Autodesk Inventor part; units mm, degrees
ref_plane "YZ Plane" through (0, 0, 0) normal (1, 0, 0) x (0, 1, 0)
ref_plane "XZ Plane" through (0, 0, 0) normal (0, 1, 0) x (-1, 0, 0)
ref_plane "XY Plane" through (0, 0, 0) normal (0, 0, 1) x (1, 0, 0)
sketch "Sketch2" plane through (0, 0, 0) normal (0, 1, 0) x (-1, 0, 0)
  line L0 (0, 0) -> (177.8, 0)
  line L1 (177.8, 0) -> (177.8, 228.6)
  line L2 (177.8, 228.6) -> (0, 228.6)
  line L3 (0, 228.6) -> (0, 0)
  dimension "d0" = 177.8
  dimension "d1" = 228.6
extrude "Extrusion1" add sketch "Sketch2" along normal blind 6.35
sketch "Sketch3" plane through (0, 6.35, 0) normal (0, 1, 0) x (1, 0, 0)
  line L0 (-177.8, -228.6) -> (0, -228.6)
  line L1 (-177.8, 0) -> (-177.8, -228.6)
  line L2 (0, 0) -> (-177.8, 0)
  line L3 (0, -228.6) -> (0, 0)
  line L4 (-88.9, -228.6) -> (-88.9, -222.25) construction
  line L5 (-88.9, 0) -> (-88.9, -6.35) construction
  line L6 (-177.8, -114.3) -> (-171.45, -114.3) construction
  line L7 (0, -114.3) -> (-6.35, -114.3) construction
  line L8 (-171.45, -114.3) -> (-171.45, -6.35)
  line L9 (-171.45, -114.3) -> (-171.45, -222.25)
  line L10 (-171.45, -6.35) -> (-88.9, -6.35)
  line L11 (-6.35, -6.35) -> (-88.9, -6.35)
  line L12 (-6.35, -6.35) -> (-6.35, -114.3)
  line L13 (-6.35, -114.3) -> (-6.35, -222.25)
  line L14 (-6.35, -222.25) -> (-88.9, -222.25)
  line L15 (-171.45, -222.25) -> (-88.9, -222.25)
  line L16 (-177.8, -228.6) -> (0, -228.6)
  line L17 (0, -228.6) -> (0, 0)
  line L18 (0, 0) -> (-177.8, 0)
  line L19 (-177.8, 0) -> (-177.8, -228.6)
  dimension "d4" = 6.35
  dimension "d5" = 6.35
  dimension "d6" = 6.35
  dimension "d7" = 6.35
extrude "Extrusion2" add sketch "Sketch3" along normal blind 38.1
sketch "Sketch4" plane through (0, 0, 0) normal (0, -1, 0) x (1, 0, 0)
  line L0 (-177.8, 0) -> (-177.8, 228.6)
  line L1 (-177.8, 228.6) -> (0, 228.6) construction
  line L2 (0, 228.6) -> (0, 0)
  line L3 (0, 0) -> (-177.8, 0)
  line L4 (-88.9, 228.6) -> (-88.9, 0) construction
  line L5 (0, 114.3) -> (-177.8, 114.3) construction
  line L6 (-88.9, 228.6) -> (-68.58, 228.6)
  line L7 (0, 228.6) -> (-177.8, 228.6) construction
  line L8 (-88.9, 228.6) -> (-109.22, 228.6)
  line L9 (-68.58, 228.6) -> (-68.58, 0) construction
  line L10 (-109.22, 228.6) -> (-109.22, 0) construction
  line L11 (-68.58, 228.6) -> (-68.58, 177.8) construction
  line L12 (-109.22, 228.6) -> (-109.22, 177.8) construction
  line L13 (-68.58, 177.8) -> (-68.58, 187.325) construction
  line L14 (-68.58, 177.8) -> (-68.58, 168.275) construction
  circle A0 centre (-68.58, 187.325) radius 2.413
  circle A1 centre (-68.58, 168.275) radius 2.413
  line L15 (-68.58, 187.325) -> (0, 187.325) construction
  line L16 (0, 187.325) -> (-12.7, 187.325) construction
  line L17 (-68.58, 168.275) -> (0, 168.275) construction
  line L18 (0, 168.275) -> (-12.7, 168.275) construction
  circle A2 centre (-12.7, 187.325) radius 2.413
  circle A3 centre (-12.7, 168.275) radius 2.413
  circle A4 centre (-68.58, 215.9) radius 2.413
  circle A5 centre (-109.22, 187.325) radius 2.413
  circle A6 centre (-109.22, 168.275) radius 2.413
  circle A7 centre (-165.1, 187.325) radius 2.413
  circle A8 centre (-165.1, 168.275) radius 2.413
  circle A9 centre (-109.22, 215.9) radius 2.413
  circle A10 centre (-68.58, 41.275) radius 2.413
  circle A11 centre (-68.58, 60.325) radius 2.413
  circle A12 centre (-12.7, 41.275) radius 2.413
  circle A13 centre (-12.7, 60.325) radius 2.413
  circle A14 centre (-68.58, 12.7) radius 2.413
  circle A15 centre (-109.22, 12.7) radius 2.413
  circle A16 centre (-109.22, 41.275) radius 2.413
  circle A17 centre (-165.1, 41.275) radius 2.413
  circle A18 centre (-165.1, 60.325) radius 2.413
  circle A19 centre (-109.22, 60.325) radius 2.413
  dimension "d10" = 20.32
  dimension "d11" = 50.8
  dimension "d12" = 9.525
  dimension "d13" = 4.826
  dimension "d14" = 4.826
  dimension "d16" = 12.7
  dimension "d17" = 4.826
  dimension "d18" = 4.826
  dimension "d19" = 12.7
  dimension "d20" = 4.826
  dimension "d21" = 12.7
extrude "Extrusion3" cut sketch "Sketch4" against normal through all
sketch "Sketch5" plane through (0, 6.35, 0) normal (0, 1, 0) x (1, 0, 0)
  circle A0 centre (-109.22, -187.325) radius 2.413
  circle A1 centre (-68.58, -168.275) radius 2.413
  circle A2 centre (-12.7, -60.325) radius 2.413
  circle A3 centre (-68.58, -12.7) radius 2.413
  circle A4 centre (-165.1, -60.325) radius 2.413
  circle A5 centre (-109.22, -60.325) radius 2.413
  circle A6 centre (-68.58, -60.325) radius 2.413
  circle A7 centre (-12.7, -168.275) radius 2.413
  circle A8 centre (-109.22, -168.275) radius 2.413
  circle A9 centre (-109.22, -215.9) radius 2.413
  circle A10 centre (-165.1, -187.325) radius 2.413
  circle A11 centre (-68.58, -187.325) radius 2.413
  circle A12 centre (-12.7, -41.275) radius 2.413
  circle A13 centre (-109.22, -12.7) radius 2.413
  circle A14 centre (-165.1, -41.275) radius 2.413
  circle A15 centre (-109.22, -41.275) radius 2.413
  circle A16 centre (-68.58, -41.275) radius 2.413
  circle A17 centre (-12.7, -187.325) radius 2.413
  circle A18 centre (-165.1, -168.275) radius 2.413
  circle A19 centre (-68.58, -215.9) radius 2.413
  line L0 (-171.45, -222.25) -> (-6.35, -222.25)
  line L1 (-6.35, -222.25) -> (-6.35, -6.35)
  line L2 (-6.35, -6.35) -> (-171.45, -6.35)
  line L3 (-171.45, -6.35) -> (-171.45, -222.25)
  line L4 (-171.45, -114.3) -> (-6.35, -114.3) construction
  line L5 (-88.9, -6.35) -> (-88.9, -222.25) construction
  line L6 (-34.925, -168.275) -> (-142.875, -168.275) construction
  line L7 (-142.875, -168.275) -> (-142.875, -60.325) construction
  line L8 (-142.875, -60.325) -> (-34.925, -60.325) construction
  line L9 (-34.925, -60.325) -> (-34.925, -168.275) construction
  line L10 (-34.925, -168.275) -> (-142.875, -60.325) construction
  line L11 (-142.875, -168.275) -> (-34.925, -60.325) construction
  circle A20 centre (-88.9, -168.275) radius 2.413
  circle A21 centre (-142.875, -114.3) radius 2.413
  circle A22 centre (-88.9, -60.325) radius 2.413
  circle A23 centre (-34.925, -114.3) radius 2.413
  point P0 (0, 0)
  point P1 (-88.9, -114.3)
  dimension "d24" = 107.95
  dimension "d25" = 107.95
  dimension "d26" = 4.826
  dimension "d27" = 4.826
  dimension "d28" = 4.826
  dimension "d29" = 4.826
extrude "Extrusion4" cut sketch "Sketch5" against normal blind 6.35 contours A20 | A21 | A22 | A23
sketch "Sketch8" plane through (0, 6.35, 0) normal (0, 1, 0) x (1, 0, 0)
  circle A0 centre (-88.9, -168.275) radius 2.413
  circle A1 centre (-88.9, -60.325) radius 2.413
  circle A2 centre (-34.925, -114.3) radius 2.413
  circle A3 centre (-142.875, -114.3) radius 2.413
  circle A4 centre (-109.22, -187.325) radius 2.413
  circle A5 centre (-68.58, -168.275) radius 2.413
  circle A6 centre (-12.7, -60.325) radius 2.413
  circle A7 centre (-68.58, -12.7) radius 2.413
  circle A8 centre (-165.1, -60.325) radius 2.413
  circle A9 centre (-109.22, -60.325) radius 2.413
  circle A10 centre (-68.58, -60.325) radius 2.413
  circle A11 centre (-12.7, -168.275) radius 2.413
  circle A12 centre (-109.22, -168.275) radius 2.413
  circle A13 centre (-109.22, -215.9) radius 2.413
  circle A14 centre (-165.1, -187.325) radius 2.413
  circle A15 centre (-68.58, -187.325) radius 2.413
  circle A16 centre (-12.7, -41.275) radius 2.413
  circle A17 centre (-109.22, -12.7) radius 2.413
  circle A18 centre (-165.1, -41.275) radius 2.413
  circle A19 centre (-109.22, -41.275) radius 2.413
  circle A20 centre (-68.58, -41.275) radius 2.413
  circle A21 centre (-12.7, -187.325) radius 2.413
  circle A22 centre (-165.1, -168.275) radius 2.413
  circle A23 centre (-68.58, -215.9) radius 2.413
  line L0 (-171.45, -222.25) -> (-6.35, -222.25)
  line L1 (-6.35, -222.25) -> (-6.35, -6.35)
  line L2 (-6.35, -6.35) -> (-171.45, -6.35)
  line L3 (-171.45, -6.35) -> (-171.45, -222.25)
  line L4 (-142.875, -114.3) -> (-34.925, -114.3) construction
  line L5 (-88.9, -60.325) -> (-88.9, -168.275) construction
  line L6 (-114.3, -88.9) -> (-63.5, -88.9) construction
  line L7 (-63.5, -88.9) -> (-63.5, -139.7) construction
  line L8 (-63.5, -139.7) -> (-114.3, -139.7) construction
  line L9 (-114.3, -139.7) -> (-114.3, -88.9) construction
  line L10 (-114.3, -88.9) -> (-63.5, -139.7) construction
  line L11 (-63.5, -88.9) -> (-114.3, -139.7) construction
  circle A24 centre (-114.3, -88.9) radius 2.413
  circle A25 centre (-63.5, -88.9) radius 2.413
  circle A26 centre (-114.3, -139.7) radius 2.413
  circle A27 centre (-63.5, -139.7) radius 2.413
  point P0 (0, 0)
  point P1 (-88.9, -114.3)
  dimension "d38" = 50.8
  dimension "d39" = 50.8
  dimension "d40" = 4.826
  dimension "d41" = 4.826
  dimension "d42" = 4.826
  dimension "d43" = 4.826
extrude "Extrusion7" cut sketch "Sketch8" against normal through all contours A24 | A25 | A26 | A27
sketch "Sketch9" plane through (-177.8, 0, 228.6) normal (0, 0, 1) x (1, 0, 0)
  line L0 (177.8, 44.45) -> (0, 44.45)
  line L1 (88.9, 44.45) -> (88.9, 0) construction
  line L2 (91.313, 0) -> (86.487, 0)
  line L3 (177.8, 0) -> (177.8, 44.45)
  line L4 (0, 0) -> (0, 44.45)
  line L5 (177.8, 22.225) -> (0, 22.225) construction
  line L6 (67.31, 9.525) -> (110.49, 9.525)
  line L7 (110.49, 9.525) -> (110.49, 34.925)
  line L8 (110.49, 34.925) -> (67.31, 34.925)
  line L9 (67.31, 34.925) -> (67.31, 9.525)
  line L10 (67.31, 9.525) -> (110.49, 34.925) construction
  line L11 (110.49, 9.525) -> (67.31, 34.925) construction
  point P0 (88.9, 22.225)
  dimension "d46" = 43.18
  dimension "d47" = 25.4
extrude "Extrusion8" cut sketch "Sketch9" against normal through all
sketch "Sketch10" plane through (0, 0, 228.6) normal (1, 0, 0) x (0, 0, -1)
  line L0 (0, 0) -> (228.6, 0)
  line L1 (228.6, 0) -> (228.6, 44.45)
  line L2 (0, 44.45) -> (228.6, 44.45)
  line L3 (0, 0) -> (0, 44.45)
  line L4 (0, 22.225) -> (228.6, 22.225) construction
  line L5 (114.3, 44.45) -> (114.3, 0) construction
  line L6 (92.71, 9.525) -> (135.89, 9.525)
  line L7 (135.89, 9.525) -> (135.89, 34.925)
  line L8 (135.89, 34.925) -> (92.71, 34.925)
  line L9 (92.71, 34.925) -> (92.71, 9.525)
  line L10 (92.71, 9.525) -> (135.89, 34.925) construction
  line L11 (135.89, 9.525) -> (92.71, 34.925) construction
  point P0 (114.3, 22.225)
  dimension "d50" = 43.18
  dimension "d51" = 25.4
extrude "Extrusion9" cut sketch "Sketch10" against normal through all contours L9 L8 L7 L6
sketch "Sketch11" plane through (-177.8, 0, 228.6) normal (0, 0, 1) x (1, 0, 0)
  line L0 (67.31, 34.925) -> (110.49, 34.925)
  line L1 (110.49, 34.925) -> (110.49, 9.525)
  line L2 (110.49, 9.525) -> (67.31, 9.525)
  line L3 (67.31, 9.525) -> (67.31, 34.925)
  line L4 (0, 0) -> (177.8, 0)
  line L5 (177.8, 0) -> (177.8, 44.45)
  line L6 (0, 44.45) -> (177.8, 44.45)
  line L7 (0, 0) -> (0, 44.45)
  point P0 (177.8, 0)
extrude "Extrusion10" add sketch "Sketch11" along normal blind 2.54
sketch "Sketch12" plane through (0, 0, 0) normal (1, 0, 0) x (0, 0, -1)
  line L0 (-135.89, 34.925) -> (-92.71, 34.925)
  line L1 (-92.71, 34.925) -> (-92.71, 9.525)
  line L2 (-92.71, 9.525) -> (-135.89, 9.525)
  line L3 (-135.89, 9.525) -> (-135.89, 34.925)
  line L4 (0, 0) -> (-231.14, 0)
  line L5 (0, 0) -> (0, 44.45)
  line L6 (0, 44.45) -> (-231.14, 44.45)
  line L7 (-231.14, 0) -> (-231.14, 44.45)
  line L8 (0, 34.925) -> (0, 9.525)
  line L9 (0, 9.525) -> (0, 34.925)
  line L10 (0, 0) -> (0, 44.45)
  line L11 (0, 0) -> (0, 44.45)
extrude "Extrusion11" add sketch "Sketch12" along normal blind 2.54
sketch "Sketch13" plane through (-177.8, 0, 0) normal (0, 0, -1) x (-1, 0, 0)
  line L0 (-110.49, 34.925) -> (-67.31, 34.925)
  line L1 (-67.31, 34.925) -> (-67.31, 9.525)
  line L2 (-67.31, 9.525) -> (-110.49, 9.525)
  line L3 (-110.49, 9.525) -> (-110.49, 34.925)
  line L4 (0, 0) -> (-180.34, 0)
  line L5 (0, 0) -> (0, 44.45)
  line L6 (0, 44.45) -> (-180.34, 44.45)
  line L7 (-180.34, 0) -> (-180.34, 44.45)
  point P0 (-177.8, 0)
extrude "Extrusion12" add sketch "Sketch13" along normal blind 2.54
sketch "Sketch14" plane through (-177.8, 0, 231.14) normal (-1, 0, 0) x (0, 0, 1)
  line L0 (-138.43, 34.925) -> (-95.25, 34.925)
  line L1 (-95.25, 34.925) -> (-95.25, 9.525)
  line L2 (-95.25, 9.525) -> (-138.43, 9.525)
  line L3 (-138.43, 9.525) -> (-138.43, 34.925)
  line L4 (-233.68, 0) -> (0, 0)
  line L5 (0, 44.45) -> (0, 0)
  line L6 (0, 44.45) -> (-233.68, 44.45)
  line L7 (-233.68, 0) -> (-233.68, 44.45)
  point P0 (-231.14, 0)
extrude "Extrusion13" add sketch "Sketch14" along normal blind 2.54
fillet "Fillet1" radius 5.08 1 edges at (-180.34, 22.225, 231.14)
fillet "Fillet2" radius 5.08 1 edges at (2.54, 22.225, -2.54)
fillet "Fillet3" radius 5.08 1 edges at (2.54, 22.225, 231.14)
fillet "Fillet4" radius 5.08 1 edges at (-180.34, 22.225, -2.54)
fillet "Fillet5" radius 3.175 4 edges at (-88.9, 44.45, -2.54) (2.54, 44.45, 114.3) (-88.9, 44.45, 231.14) (-180.34, 44.45, 114.3)
equation "\"d2\" = base_thickness"
equation "\"d4\" = base_thickness"
equation "\"d5\" = base_thickness"
equation "\"d6\" = base_thickness"
equation "\"d7\" = base_thickness"
equation "\"d10\" = motor_adapter_across"
equation "\"d12\" = 0.5 * motor_adapter_width"
equation "\"d19\" = d16"
equation "\"d21\" = d16"
equation "\"base_thickness\" = 6.35"
equation "\"motor_adapter_width\" = 19.05"
equation "\"motor_adapter_across\" = 20.32"
properties part number "base"
Source: CAD feature listing. Evaluate the final solid. Frame: model axes, mm. A direction names the side the tool comes from. Round coordinates to 2 decimals unless told otherwise and drop trailing zeros. Loops run counter-clockwise (first coordinate to the right, second up) from the corner with the lowest first, then second, coordinate; pieces in that order, holes last. Notation, with made-up numbers: (-24.5, -8.75) -> (20.5, -8.75) arc R14 cw to (20.5, -1.75) -> close; hole circle Ø10 at (55.5, 63.25). An arc over 180 degrees is marked (long way). Answer as a JSON object with one key per item and string values. Group by question number.
Q1. Section query B-B (z = 114.3). Output: boundary loops of the cut face in (x, y) (3 decimals).
Q2. Section query A-A (x = -12.7). Output: boundary loops of the cut face in (y, z) (3 decimals), plus the area to 3 significant figures.
Q3. Access query for faces 1 (the flat face through (-2, 22, 135.89)), 2 (the cylindrical face through (-86.67, 3.22, 61.25)), 3 (the flat face through (-171.45, 38, 113)). Directions: +Z, -Z, +X, -X, +Y, -Y. A direction counts if a zero-diameter tool reaches every point of the face in a straight line with its end or side. Return the directions, or none.
Q4. Section query D-D (z = 88.9). Output: boundary loops of the cut face in (x, y) (3 decimals).
Q5. Ray query, line 1 (Z direction, x = -63, y = 4); line 2 (Z direction, x = -88.9, y = 3); line 3 (X direction, y = 10, z = 164). Return the intervals inside material, ascending. Write a range as from..to.
Q6. Section query C-C (y = 21). Output: boundary loops of the cut face in (x, z).
Q7. Contact query for flat-ended pins moving along their axis: P1, Ø7.5, axis at x = -63.5, z = 139.7, coming from the +Y side; P2, Ø5, axis at x = -79, z = 128, coming from the -Y side. Output: stop coordinate, or through.
Q8. Mould query, pull axis X, two halves, no side actions, for faces 4 (the cylindrical face through (-70.495, 3.131, 11.232)), 5 (the flat face through (-2, 9.525, 114)). Classes: pulls with the +X half, pulls with the -X half, needs draft (parallel to the pull), parting line crosses it, or undercut.
Completed:
{
 "1": {"outline": "(-180.34, 0) -> (-145.288, 0) -> (-145.288, 6.35) -> (-171.45, 6.35) -> (-171.45, 9.525) -> (-180.34, 9.525) -> close; (-180.34, 34.925) -> (-171.45, 34.925) -> (-171.45, 44.45) -> (-177.165, 44.45) arc R3.175 ccw to (-180.34, 41.275) -> close; (-140.462, 0) -> (-37.338, 0) -> (-37.338, 6.35) -> (-140.462, 6.35) -> close; (-32.512, 0) -> (2.54, 0) -> (2.54, 9.525) -> (-6.35, 9.525) -> (-6.35, 6.35) -> (-32.512, 6.35) -> close; (-6.35, 34.925) -> (2.54, 34.925) -> (2.54, 41.275) arc R3.175 ccw to (-0.635, 44.45) -> (-6.35, 44.45) -> close"},
 "2": {"outline": "(0, -2.54) -> (41.275, -2.54) arc R3.175 ccw to (44.45, 0.635) -> (44.45, 6.35) -> (6.35, 6.35) -> (6.35, 38.862) -> (0, 38.862) -> close; (0, 43.688) -> (6.35, 43.688) -> (6.35, 57.912) -> (0, 57.912) -> close; (0, 62.738) -> (6.35, 62.738) -> (6.35, 165.862) -> (0, 165.862) -> close; (0, 170.688) -> (6.35, 170.688) -> (6.35, 184.912) -> (0, 184.912) -> close; (0, 189.738) -> (6.35, 189.738) -> (6.35, 222.25) -> (44.45, 222.25) -> (44.45, 227.965) arc R3.175 ccw to (41.275, 231.14) -> (0, 231.14) -> close", "area": "2,030 mm²"},
 "3": {"face 1": "+X, -X", "face 2": "+Y, -Y", "face 3": "+Y"},
 "4": {"outline": "(-180.34, 0) -> (-116.713, 0) -> (-116.713, 6.35) -> (-171.45, 6.35) -> (-171.45, 44.45) -> (-177.165, 44.45) arc R3.175 ccw to (-180.34, 41.275) -> close; (-111.887, 0) -> (-65.913, 0) -> (-65.913, 6.35) -> (-111.887, 6.35) -> close; (-61.087, 0) -> (2.54, 0) -> (2.54, 41.275) arc R3.175 ccw to (-0.635, 44.45) -> (-6.35, 44.45) -> (-6.35, 6.35) -> (-61.087, 6.35) -> close"},
 "5": {"line 1": "-2.54..86.54, 91.26..137.34, 142.06..231.14", "line 2": "-2.54..57.91, 62.74..165.86, 170.69..231.14", "line 3": "-180.34..-171.45, -6.35..2.54"},
 "6": {"outline": "(-180.34, 2.54) arc R5.08 ccw to (-175.26, -2.54) -> (-110.49, -2.54) -> (-110.49, 6.35) -> (-171.45, 6.35) -> (-171.45, 92.71) -> (-180.34, 92.71) -> close; (-180.34, 135.89) -> (-171.45, 135.89) -> (-171.45, 222.25) -> (-110.49, 222.25) -> (-110.49, 231.14) -> (-175.26, 231.14) arc R5.08 ccw to (-180.34, 226.06) -> close; (-67.31, -2.54) -> (-2.54, -2.54) arc R5.08 ccw to (2.54, 2.54) -> (2.54, 92.71) -> (-6.35, 92.71) -> (-6.35, 6.35) -> (-67.31, 6.35) -> close; (-67.31, 222.25) -> (-6.35, 222.25) -> (-6.35, 135.89) -> (2.54, 135.89) -> (2.54, 226.06) arc R5.08 ccw to (-2.54, 231.14) -> (-67.31, 231.14) -> close"},
 "7": {"P1": "y = 6.35", "P2": "y = 0"},
 "8": {"face 4": "undercut", "face 5": "needs draft"}
}
